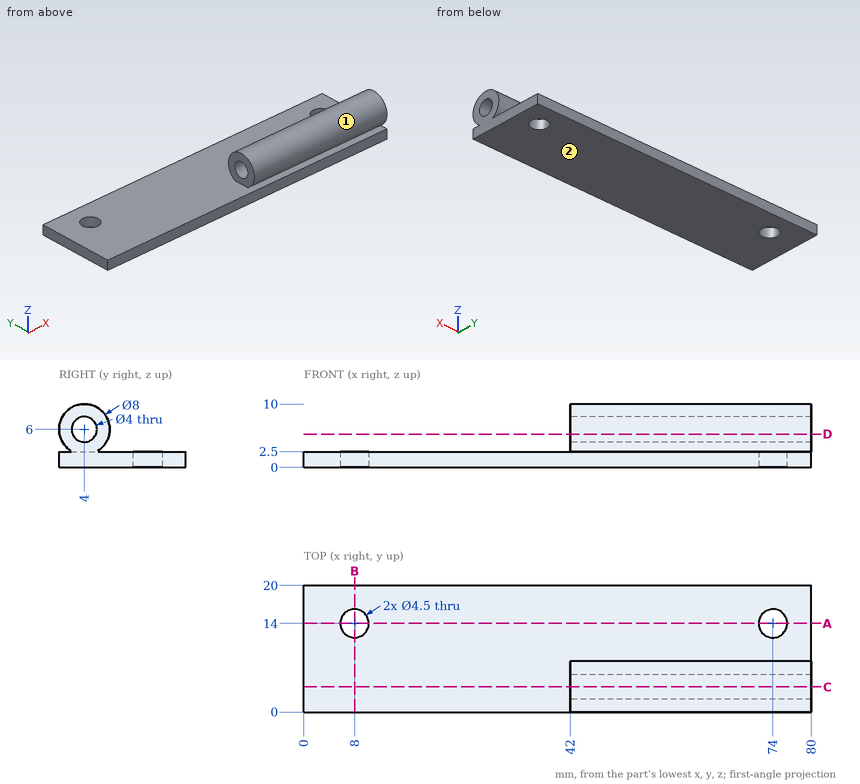
Verification items for this drawing (mm, ordinates from the low corner). Round coordinates to 2 decimals unless told otherwise and drop trailing zeros. Loops run counter-clockwise (first coordinate to the right, second up) from the corner with the lowest first, then second, coordinate; pieces in that order, holes last. Notation, with made-up numbers: (-25.5, 39.5) -> (-18.5, 39.5) arc R35 cw to (-18.5, 78.5) -> close; hole circle Ø4 at (-21.75, 73.5). An arc over 180 degrees is marked (long way). Write item = value, one per line. Start each with the question number.
1) Sectioned sample at A-A, the plane y = 14. Record the cut outline in (x, z), plus the area to 4 significant figures.
2) Gauge pin test, flat ends, axial feed: pin 1 Ø10 at (x, y) = (26.5, 13) entering from +Z; pin 2 Ø5 at (x, z) = (47.5, 8.5) entering from +Y; pin 3 Ø3 at (y, z) = (18, 5.5) entering from -X; pin 4 Ø1 at (y, z) = (3.5, 4.5) entering from -X. Record the tip position at first contact, or that the pin passes through.
3) Thickness scan on probe 1 along Y at (x, z) = (75, 5.75); probe 2 along Y at (x, z) = (74, 0.75); probe 3 along Z at (x, y) = (7, 4). Record the ranges inside material, lowest first.
4) Sectioned sample at C-C, the plane y = 4. Record the cut outline in (x, z).
5) Sectioned sample at D-D, the plane z = 5.25. Record the cut outline in (x, y).
6) Release check for a two-part mould opening along Z. For the marked faces 1 and 2 record: released by +Z, released by -Z, zero draft, split by the parting line, or undercut.
7) Sectioned sample at B-B, the plane x = 8. Record the cut outline in (y, z), plus the area to 4 significant figures.
Results are:
q1.outline = (0, 0) -> (5.75, 0) -> (5.75, 2.5) -> (0, 2.5) -> close; (10.25, 0) -> (71.75, 0) -> (71.75, 2.5) -> (10.25, 2.5) -> close; (76.25, 0) -> (80, 0) -> (80, 2.5) -> (76.25, 2.5) -> close
q1.area = 177.5 mm^2
q2.pin_1 = 2.5
q2.pin_2 = 8
q2.pin_3 = through
q2.pin_4 = 42
q3.probe_1 = 0.01 to 2.02, 5.98 to 7.99
q3.probe_2 = 0 to 11.75, 16.25 to 20
q3.probe_3 = 0 to 2.5
q4.outline = (0, 0) -> (80, 0) -> (80, 4) -> (42, 4) -> (42, 2.5) -> (0, 2.5) -> close; (42, 8) -> (80, 8) -> (80, 10) -> (42, 10) -> close
q5.outline = (42, 0.07) -> (80, 0.07) -> (80, 2.15) -> (42, 2.15) -> close; (42, 5.85) -> (80, 5.85) -> (80, 7.93) -> (42, 7.93) -> close
q6.face_1 = undercut
q6.face_2 = released by -Z
q7.outline = (0, 0) -> (11.75, 0) -> (11.75, 2.5) -> (0, 2.5) -> close; (16.25, 0) -> (20, 0) -> (20, 2.5) -> (16.25, 2.5) -> close
q7.area = 38.75 mm^2
